The figure shows three views and two pictorial views of one solid part (mm, origin at its lowest corner). Answer the questions. A direction names the side the tool comes from. Coordinates: 2 decimals unless noted, no trailing zeros. Write each loop counter-clockwise with the first axis right and the second up, starting at its lowest first coordinate (ties: lowest second). Pieces come first, ordered by that corner, then holes.
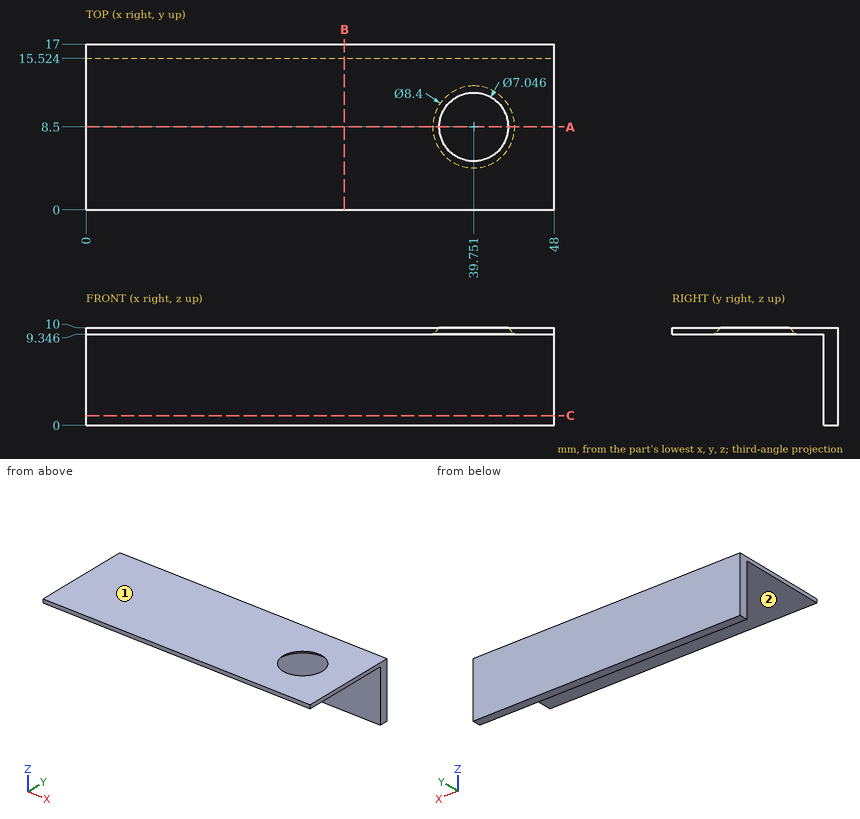
Q1. Which of the six approach directions +Z, -Z, +X, -X, +Y, -Y give full straight-line access (tool end or side, diameter ignored) to the marked faces 1 and 2?
Answers below:
face 1: +Z, +X, -X, +Y, -Y
face 2: -Z, +X, -X, -Y
Q2. The part is cut by section C-C, the plane z = 1. Write down the section's boundary in (x, y).
Answers below:
outline: (0, 15.52) - (48, 15.52) - (48, 17) - (0, 17) - close
Q3. Given pin 1 (4 mm diameter, centred on x = 37.5, z = 7.5, fed in from -Y); pin 2 (8 mm diameter, centred on x = 30, y = 6.5, fed in from -Z); pin 3 (1.5 mm diameter, centred on x = 13.5, z = 8, fed in from -Y), each flat-ended and moving along its own axis, determine where each tip first touches the part or whether it passes through.
Answers below:
pin 1: stops at y = 0
pin 2: stops at z = 9.35
pin 3: stops at y = 15.52
Q4. The part is cut by section A-A, the plane y = 8.5. Write down the section's boundary in (x, z).
Answers below:
outline: (0, 9.35) - (35.55, 9.35) - (36.23, 10) - (0, 10) - close; (43.27, 10) - (43.95, 9.35) - (48, 9.35) - (48, 10) - close
Q5. Find the intervals of material crossed by probe 1 along Z at (x, y) = (21.5, 2.25); probe 2 along Y at (x, z) = (10.5, 6.5), in increasing order.
Answers below:
probe 1: z = 9.35 to 10
probe 2: y = 15.52 to 17
Q6. The part is cut by section B-B, the plane x = 26.5. Write down the section's boundary in (y, z).
Answers below:
outline: (0, 9.35) - (15.52, 9.35) - (15.52, 0) - (17, 0) - (17, 10) - (0, 10) - close
